Input: part model. Units: mm. Frame: model coordinates. A direction names the side the tool comes from. Round coordinates to 2 decimals unless told otherwise and drop trailing zeros. Loops run counter-clockwise (first coordinate to the right, second up) from the corner with the lowest first, then second, coordinate; pieces in that order, holes last. Notation, with made-up numbers: M -24,71 L 13,71 A19 ccw 13,94 Z; hole C 52,77 d4. An arc over 180 degrees is marked long. Return JSON: item names as keys, results as strings. Group by question number.
1) Section B-B (z = 3.65). Output: boundary loops of the cut face in (x, y).
2) Material intervals for line 1 (Y direction, x = 15, z = 2.3); line 2 (Y direction, x = 13, z = 2.2); line 3 (X direction, y = -11, z = 1.5), sorted ascending. Write a range as from..to.
3) Mould query, pull axis X, two halves, no side actions, for faces 1 (the face through (15.07, 12.6, 2.79)), 2 (the face through (34.43, 7.6, 2.71)), 3 (the face through (-34.4, 14.43, 2.79)), 4 (the face through (0, -15, 3)). Classes: +X half, -X half, draft (parallel to the pull), parting line (faces both ways), or undercut.
4) Access query for faces 5 (the face through (35, -11, 3)), 6 (the face through (34.4, -7.57, 2.71)). Directions: +Z, -Z, +X, -X, +Y, -Y. A direction counts if a zero-diameter tool reaches every point of the face in a straight line with its end or side. Return the directions, or none.
5) Section C-C (y = -11). Output: boundary loops of the cut face in (x, z), plus the area to 3 significant figures.
6) Section A-A (x = 2.5). Output: boundary loops of the cut face in (y, z).
7) Contact query for flat-ended pins moving along their axis: P1, Ø3, axis at x = 15, y = 11, coming from the +Z side; P2, Ø3, axis at y = -6, z = 4, coming from the +X side. Output: stop coordinate, or through.
8) Section D-D (x = 15). Output: boundary loops of the cut face in (y, z).
Solid Edge part; units mm, degrees
sketch "Sketch1" plane through (0, 0, 0) normal (0, 0, 1) x (1, 0, 0)
  line L0 (35, -15) -> (-35, -15)
  line L1 (-35, -15) -> (-35, 15)
  line L2 (-35, 15) -> (35, 15)
  line L3 (35, 15) -> (35, -15)
  dimension "D1" = 35
  dimension "D2" = 35
  dimension "D3" = 35
extrude "Protrusion1" add sketch "Sketch1" along normal blind 5.5
sketch "Sketch2" plane through (0, 0, 5.5) normal (0, 0, 1) x (1, 0, 0)
  line L0 (35, 7) -> (-27, 7)
  line L1 (-27, 7) -> (-27, -7)
  line L2 (-27, -7) -> (35, -7)
  line L3 (35, -7) -> (35, 7)
  dimension "D1" = 35
  dimension "D2" = 27
extrude "Cutout1" cut sketch "Sketch2" against normal through all
hole "Hole_1" at (15, 11, 5.5) direction (0, 0, -1) diameter 3.2 end up to next
hole "Hole1" at (15, -11, 5.5) direction (0, 0, -1) diameter 3.2 end up to next
fillet "Round_1" radius 2 6 edges at (-35, -15, 2.75) (35, -15, 2.75) (35, -7, 2.75) (35, 7, 2.75) (35, 15, 2.75) (-35, 15, 2.75)
properties material "木材, アッシュ"
Returned:
{
 "1": {"outline": "M -35,-13 A2 ccw -33,-15 L 33,-15 A2 ccw 35,-13 L 35,-9 A2 ccw 33,-7 L -27,-7 L -27,7 L 33,7 A2 ccw 35,9 L 35,13 A2 ccw 33,15 L -33,15 A2 ccw -35,13 Z; hole C 15,-11 d3.2; hole C 15,11 d3.2"},
 "2": {"line 1": "y = -15..-12.6, -9.4..-7, 7..9.4, 12.6..15", "line 2": "y = -15..-7, 7..15", "line 3": "x = -35..13.4, 16.6..35"},
 "3": {"face 1": "undercut", "face 2": "+X half", "face 3": "-X half", "face 4": "draft"},
 "4": {"face 5": "+Z, -Z, +X, +Y, -Y", "face 6": "+Z, -Z, +X"},
 "5": {"outline": "M -35,0 L 13.4,0 L 13.4,5.5 L -35,5.5 Z; M 16.6,0 L 35,0 L 35,5.5 L 16.6,5.5 Z", "area": "367 mm^2"},
 "6": {"outline": "M -15,0 L -7,0 L -7,5.5 L -15,5.5 Z; M 7,0 L 15,0 L 15,5.5 L 7,5.5 Z"},
 "7": {"P1": "passes through", "P2": "stops at x = 34.32"},
 "8": {"outline": "M -15,0 L -12.6,0 L -12.6,5.5 L -15,5.5 Z; M -9.4,0 L -7,0 L -7,5.5 L -9.4,5.5 Z; M 7,0 L 9.4,0 L 9.4,5.5 L 7,5.5 Z; M 12.6,0 L 15,0 L 15,5.5 L 12.6,5.5 Z"}
}
